Autodesk Inventor part; units mm, degrees
ref_plane "YZ Plane" through (0, 0, 0) normal (1, 0, 0) x (0, 1, 0)
ref_plane "XZ Plane" through (0, 0, 0) normal (0, 1, 0) x (-1, 0, 0)
ref_plane "XY Plane" through (0, 0, 0) normal (0, 0, 1) x (1, 0, 0)
sketch "Sketch1" plane through (0, 0, 0) normal (0, 0, 1) x (1, 0, 0)
  line L0 (4.25, 0) -> (4.25, 4.5)
  line L1 (4.25, 4.5) -> (0, 4.5)
  line L2 (4.25, 0) -> (1.75, 0)
  line L3 (1.75, 0) -> (1.75, -34)
  line L4 (1.75, -34) -> (2.5, -34)
  line L5 (2.5, -34) -> (2.5, -40)
  line L6 (2.5, -40) -> (0, -40)
  line L7 (0, 4.5) -> (0, -40)
  point P0 (0, 0)
  dimension "d0" = 8.5
  dimension "d2" = 3.5
  dimension "d3" = 5
  dimension "d4" = 4.5
  dimension "d5" = 6
  dimension "d6" = 40
revolve "Вращение1" add sketch "Sketch1" angle 360 about axis through (0, 4.5, 0) along (0, -1, 0)
sketch "Sketch2" plane through (0, 4.5, 0) normal (0, 1, 0) x (1, 0, 0)
  circle A0 centre (0, 0) radius 4.25 construction
  circle A1 centre (0, 0) radius 1.25
  dimension "d31" = 2.5
extrude "Выдавливание1" cut sketch "Sketch2" against normal blind 1.5
chamfer "Фаска1" distance 0.9 angle 45 1 edges at (-4.25, 4.5, 0)
sketch "Sketch3" plane through (0, 0, 0) normal (0, 0, 1) x (1, 0, 0)
  line L0 (0, 0) -> (0, 4.5)
  line L1 (-2.3552, 0) -> (2.3552, 0) construction
  line L2 (-4.25, 4.5) -> (4.25, 4.5) construction
  line L3 (-0.6, 4.5) -> (0.6, 4.5)
  line L4 (0.6, 4.5) -> (0.6, 1.3)
  line L5 (0.6, 1.3) -> (-0.6, 1.3)
  line L6 (-0.6, 1.3) -> (-0.6, 4.5)
  dimension "d8" = 1.3
  dimension "d9" = 1.2
extrude "Выдавливание2" cut sketch "Sketch3" along normal through all both and the other way through all
fillet "Сопряжение1" radius 0.4 2 edges at (-1.75, 0, 0) (-1.75, -34, 0)
thread "Резьба1"
chamfer "Фаска2" distance 0.9 angle 45 1 edges at (-2.5, -40, 0)
equation "\"d31\" = d3_"
equation "\"d32\" = h3"
equation "\"d21\" = C1"
equation "\"d8\" = h2"
equation "\"d9\" = n"
equation "\"d12\" = R"
equation "\"d13\" = b"
equation "\"d15\" = C1"
equation "\"d0\" = D"
equation "\"d2\" = d1"
equation "\"d3\" = d_"
equation "\"d4\" = k1"
equation "\"d5\" = b"
equation "\"d6\" = l_"
equation "\"D\" = 8.5"
equation "\"d_\" = 5"
equation "\"l_\" = 40"
equation "\"b\" = 6"
equation "\"d1\" = 3.5"
equation "\"R\" = 0.4"
equation "\"C1\" = 0.9"
equation "\"h2\" = 1.3"
equation "\"n\" = 1.2"
equation "\"h3\" = 1.5"
equation "\"k1\" = 4.5"
equation "\"d3_\" = 2.5"
equation "\"G\" = l_ - b"
properties part number "Винт 3 M5-6gx40 ГОСТ 10336-80" material "Сталь, мягкая"
The listing builds one solid part. Answer for the finished solid, in the listing's coordinates (mm). A direction names the side the tool comes from. Give positions to 0.01 mm unless a question says otherwise; leave off trailing zeros. Order: outer loops, then holes, each group sorted by start corner. A loop starts at its lowest first (then second) coordinate and runs counter-clockwise, first axis right, second up. Notation, with made-up numbers: M -27,31 L 26,31 A16 ccw 26,54 Z; hole C 14.25,50.5 d11. An arc over 180 degrees is marked long. Put each result on its own line as item: value. Start each with the question number.
Item 1: The part is cut by section A-A, the plane x = 0. Determine the outline of the cut face in (y, z).
Item 2: The part is cut by section D-D, the plane y = -21. Determine the outline of the cut face in (x, z).
Item 3: Find the intervals of material crossed by line 1 along Y through (x, z) = (0.5, -3); line 2 along Y through (x, z) = (-1.5, -3); line 3 along X through (y, z) = (1.5, 3.75), in increasing order.
Item 4: Which of the six approach directions +Z, -Z, +X, -X, +Y, -Y give full straight-line access (tool end or side, diameter ignored) to faces 1 (the face through (-1.25, 3.76, -0.02)), 2 (the face through (1.617, -17.232, -0.67)), 3 (the face through (2, 4.5, 0)), 4 (the face through (-0.6, 2.5, -0.1)), 5 (the face through (-0.92, 1.83, 4.15))?
Item 5: The part is cut by section B-B, the plane y = 2. Determine the outline of the cut face in (x, z), and give its area (3 significant figures).
Item 6: For a pull along Z with two mould halves and no side action, classify faces 6 (the face through (2, 0, -2)), 7 (the face through (1.25, 3.76, 0.02)), 8 (the face through (-0.54, -36.59, -2.44)) as +Z half, -Z half, draft (parallel to the pull), parting line (faces both ways), or undercut.
Item 7: Flat-ended cylindrical pins translate along their axes: P1, Ø1.6, axis at y = 3.5, z = -1, coming from the +X side; P2, Ø4, axis at y = -20, z = 1, coming from the +X side; P3, Ø0.6, axis at x = 0, z = -1, coming from the +Y side. Find the tip coordinate at first contact, or state that the pin passes through.
Item 8: The part is cut by section C-C, the plane z = 0. Determine the outline of the cut face in (x, y).
Answer key:
1. outline: M -40,-1.6 L -39.1,-2.5 L -34,-2.5 L -34,-2.15 A0.4 cw -33.6,-1.75 L -0.4,-1.75 A0.4 cw 0,-2.15 L 0,-4.25 L 1.3,-4.25 L 1.3,4.25 L 0,4.25 L 0,2.15 A0.4 cw -0.4,1.75 L -33.6,1.75 A0.4 cw -34,2.15 L -34,2.5 L -39.1,2.5 L -40,1.6 Z
2. outline: C 0,0 d3.5
3. line 1: y = 0 to 1.3
3. line 2: y = 0 to 4.5
3. line 3: x = -2 to -0.6, 0.6 to 2
4. face 1: +Y
4. face 2: none
4. face 3: +Z, -Z, +X, -X, +Y
4. face 4: +Z, -Z, +Y
4. face 5: +Y, -Y
5. outline: M -0.6,-4.21 L -0.6,4.21 A4.25 ccw Z; M 0.6,-4.21 A4.25 ccw 0.6,4.21 Z
5. area: 46.6 mm²
6. face 6: draft
6. face 7: undercut
6. face 8: parting line
7. P1: stops at x = 4.25
7. P2: stops at x = 1.75
7. P3: stops at y = 1.3
8. outline: M -4.25,0 L -2.15,0 A0.4 cw -1.75,-0.4 L -1.75,-33.6 A0.4 cw -2.15,-34 L -2.5,-34 L -2.5,-39.1 L -1.6,-40 L 1.6,-40 L 2.5,-39.1 L 2.5,-34 L 2.15,-34 A0.4 cw 1.75,-33.6 L 1.75,-0.4 A0.4 cw 2.15,0 L 4.25,0 L 4.25,3.6 L 3.35,4.5 L 1.25,4.5 L 1.25,3 L 0.6,3 L 0.6,1.3 L -0.6,1.3 L -0.6,3 L -1.25,3 L -1.25,4.5 L -3.35,4.5 L -4.25,3.6 Z
